Design review of the part built by this model. Coordinates are the model's own, in mm. A direction names the side the tool comes from. Coordinates: 2 decimals unless noted, no trailing zeros. Order: outer loops, then holes, each group sorted by start corner. A loop starts at its lowest first (then second) coordinate and runs counter-clockwise, first axis right, second up. Notation, with made-up numbers: (2, 28.5) -> (51, 28.5) arc R35 cw to (51, 63.5) -> close; hole circle Ø6 at (33.5, 11). An arc over 180 degrees is marked (long way). Write item = value, one per line.
```python
from build123d import *

# Parameters (mm, degrees)
BOSS_EXTRUDE1_DEPTH     = 1.9
SKETCH2_R               = 3.55
SKETCH2_R_2             = 2.45
BOSS_EXTRUDE2_DEPTH     = 2
CUT_EXTRUDE1_START      = -2.5
SKETCH3_R               = 2.45
CUT_EXTRUDE1_DEPTH      = 2.5
CUT_EXTRUDE2_DEPTH      = 14.232630124
CUT_EXTRUDE2_DEPTH_BACK = 14.232630124
SKETCH4_R               = 0.468509015
SKETCH4_R_2             = 0.881877008


with BuildPart() as part:
    # Sketch1 → Boss-Extrude1 (new body)
    with BuildSketch(Plane(origin=(0, 0, 0), x_dir=(1, 0, 0), z_dir=(0, 1, 0))):
        with BuildLine():
            Line((-3.487806971, 0.661590909), (-1.473721255, 11.279545455))
            ThreePointArc((-1.473721255, 11.279545455), (0, 12.5), (1.473721255, 11.279545455))
            Line((1.473721255, 11.279545455), (3.487806971, 0.661590909))
            ThreePointArc((3.487806971, 0.661590909), (0, -3.55), (-3.487806971, 0.661590909))
        make_face()
    extrude(amount=BOSS_EXTRUDE1_DEPTH)

    # Sketch2 → Boss-Extrude2 (add)
    with BuildSketch(Plane(origin=(0, 1.9, 0), x_dir=(1, 0, 0), z_dir=(0, 1, 0))):
        with Locations(Location((0, 0, 0), (0, 0, 10.740645756))):
            Circle(SKETCH2_R)
        with Locations(Location((0, 0, 0), (0, 0, 270))):
            Circle(SKETCH2_R_2, mode=Mode.SUBTRACT)
    extrude(amount=BOSS_EXTRUDE2_DEPTH)

    # Sketch3 → Cut-Extrude1 (cut)
    with BuildSketch(Plane(origin=(0, 3.9, 0), x_dir=(1, 0, 0), z_dir=(0, 1, 0)).offset(CUT_EXTRUDE1_START)):
        with Locations(Location((0, 0, 0), (0, 0, 270))):
            Circle(SKETCH3_R)
    extrude(amount=CUT_EXTRUDE1_DEPTH, mode=Mode.SUBTRACT)

    # Sketch4 → Cut-Extrude2 (cut, two sides: drawn at the far end of the back side and taken through both)
    with BuildSketch(Plane(origin=(0, 1.4, 0), x_dir=(1, 0, 0), z_dir=(0, 1, 0)).offset(-CUT_EXTRUDE2_DEPTH_BACK)):
        with Locations(Location((0, 11, 0), (0, 0, 270))):
            Circle(SKETCH4_R)
        with Locations(Location((0, 0, 0), (0, 0, 270))):
            Circle(SKETCH4_R_2)
    extrude(amount=CUT_EXTRUDE2_DEPTH + CUT_EXTRUDE2_DEPTH_BACK, mode=Mode.SUBTRACT)


solid = part.part
```
(1) We need section B-B (z = 0). Write out the cut boundary in (x, y), and give its area (3 significant figures).
Report:
outline = (-3.55, 0) -> (-0.88, 0) -> (-0.88, 1.4) -> (-2.45, 1.4) -> (-2.45, 3.9) -> (-3.55, 3.9) -> close; (0.88, 0) -> (3.55, 0) -> (3.55, 3.9) -> (2.45, 3.9) -> (2.45, 1.4) -> (0.88, 1.4) -> close
area = 13.0 mm²
(2) We need section D-D (x = -3). Write out the cut boundary in (y, z), and give its area (3 significant figures).
Report:
outline = (0, -3.23) -> (1.9, -3.23) -> (1.9, -1.9) -> (3.9, -1.9) -> (3.9, 1.9) -> (0, 1.9) -> close
area = 17.3 mm²
(3) We need section C-C (y = 0.55). Write out the cut boundary in (x, z).
Report:
outline = (-3.49, -0.66) -> (-1.47, -11.28) arc R1.5 ccw to (1.47, -11.28) -> (3.49, -0.66) arc R3.55 ccw (long way) to start; hole circle Ø1.76 at (0, 0); hole circle Ø0.94 at (0, -11)
(4) Insertion check: pin 1 (1.1 mm diameter, centred on x = 0, z = 0, fed in from +Y); pin 2 (1 mm diameter, centred on y = 2, z = -2.5, fed in from +X); pin 3 (4 mm diameter, centred on x = 1, z = -10.5, fed in from +Y); pin 4 (1 mm diameter, centred on x = 2, y = 1, fed in from +Z). Each pin has a flat end and moves straight along its axis. Give the tip position at first contact, or say it passes through.
Report:
pin_1 = through
pin_2 = 3.23
pin_3 = 1.9
pin_4 = 3.22
(5) The part is to be moulded in two halves that separate along X. For faces 1 (the cylindrical face through (0, 0.9, -12.5)), 2 (the flat face through (0, 1.9, -7)), 3 (the cylindrical face through (0.736, 2.632, 2.337)), say which applies: released by +X, released by -X, zero draft, split by the parting line, or undercut.
Report:
face_1 = split by the parting line
face_2 = zero draft
face_3 = undercut
(6) For L1, parallel to X at y = 2, z = 0; L2, parallel to Y at x = -0.75, z = -0.75; L3, parallel to Y at x = -0.25, z = -8.5, list the stretches that pass through material, from the lowest coordinate up.
Report:
L1 = -3.55 to -2.45, 2.45 to 3.55
L2 = 0 to 1.4
L3 = 0 to 1.9
(7) For faces 4 (the flat face through (-1.1, 1.4, 0)), 5 (the flat face through (2.467, 0.937, -6.045)), list the 3-axis set-ups (+Z, -Z, +X, -X, +Y, -Y) from which the entire face can be reached by the end or side of a thin tool; tool diameter is ignored.
Report:
face_4 = +Y
face_5 = -Z, +X, +Y, -Y
(8) We need section A-A (x = 0). Write out the cut boundary in (y, z).
Report:
outline = (0, -12.5) -> (1.9, -12.5) -> (1.9, -11.47) -> (0, -11.47) -> close; (0, -10.53) -> (1.9, -10.53) -> (1.9, -3.55) -> (3.9, -3.55) -> (3.9, -2.45) -> (1.4, -2.45) -> (1.4, -0.88) -> (0, -0.88) -> close; (0, 0.88) -> (1.4, 0.88) -> (1.4, 2.45) -> (3.9, 2.45) -> (3.9, 3.55) -> (0, 3.55) -> close
